```python
from build123d import *

# Parameters (mm, degrees)
SKETCH_2_R          = 1.75
SKETCH_2_R_2        = 6
EXTRUDE_1_DEPTH     = 8
SKETCH_3_R          = 8.05
CUT_EXTRUDE_1_DEPTH = 3.5
SKETCH_4_W          = 16.75
SKETCH_4_H          = 17
EXTRUDE_2_DEPTH     = 30
SKETCH_5_R          = 1.75
CUT_EXTRUDE_2_DEPTH = 51.685920136
EXTRUDE_3_DEPTH     = 2
EXTRUDE_4_DEPTH     = 2


with BuildPart() as part:
    # 草图2 → 凸台-拉伸1 (new body)
    with BuildSketch(Plane.XY):
        with BuildLine():
            Line((-6.25, 21.25), (6.25, 21.25))
            ThreePointArc((6.25, 21.25), (9.785533906, 19.785533906), (11.25, 16.25))
            Line((11.25, 16.25), (11.25, -16.25))
            ThreePointArc((11.25, -16.25), (9.785533906, -19.785533906), (6.25, -21.25))
            Line((6.25, -21.25), (-6.25, -21.25))
            ThreePointArc((-6.25, -21.25), (-9.785533906, -19.785533906), (-11.25, -16.25))
            Line((-11.25, -16.25), (-11.25, 16.25))
            ThreePointArc((-11.25, 16.25), (-9.785533906, 19.785533906), (-6.25, 21.25))
        make_face()
        with Locations((0, -16.25)):
            Circle(SKETCH_2_R, mode=Mode.SUBTRACT)
        Circle(SKETCH_2_R_2, mode=Mode.SUBTRACT)
        with Locations((0, 16.25)):
            Circle(SKETCH_2_R, mode=Mode.SUBTRACT)
    extrude(amount=EXTRUDE_1_DEPTH)

    # 草图3 → 切除-拉伸1 (cut)
    with BuildSketch(Plane(origin=(0, 0, 0), x_dir=(-1, 0, 0), z_dir=(0, 0, -1))):
        Circle(SKETCH_3_R)
    extrude(amount=-CUT_EXTRUDE_1_DEPTH, mode=Mode.SUBTRACT)

    # 草图4 → 凸台-拉伸2 (add)
    with BuildSketch(Plane.XY):
        with Locations((-19.625, 0)):
            Rectangle(SKETCH_4_W, SKETCH_4_H)
    extrude(amount=EXTRUDE_2_DEPTH)

    # 草图5 → 切除-拉伸2 (cut, through all)
    with BuildSketch(Plane.XZ.offset(8.5)):
        with Locations(Location((-23, 22.5, 0), (0, 0, 270))):
            Circle(SKETCH_5_R)
        with Locations(Location((-23, 7.5, 0), (0, 0, 270))):
            Circle(SKETCH_5_R)
    extrude(amount=-CUT_EXTRUDE_2_DEPTH, mode=Mode.SUBTRACT)

    # 草图7 → 凸台-拉伸3 (add)
    with BuildSketch(Plane.XZ.offset(8.5)):
        Polygon((-11.25, 20), (-11.25, 8), (-4.32179677, 8), align=None)
    extrude(amount=-EXTRUDE_3_DEPTH)

    # 草图8 → 凸台-拉伸4 (add)
    with BuildSketch(Plane(origin=(0, 8.5, 0), x_dir=(1, 0, 0), z_dir=(0, 1, 0))):
        Polygon((-4.32179677, -8), (-11.25, -20), (-11.25, -8), align=None)
    extrude(amount=-EXTRUDE_4_DEPTH)


solid = part.part
```
Can you work these out from the model? Positions are in its coordinate system, mm. A direction names the side the tool comes from. Coordinates: 2 decimals unless noted, no trailing zeros. Write each loop counter-clockwise with the first axis right and the second up, starting at its lowest first coordinate (ties: lowest second). Pieces come first, ordered by that corner, then holes. Notation, with made-up numbers: M 84.5,28 L 138.5,28 A20 cw 138.5,33 Z; hole C 80.25,74.5 d11. An arc over 180 degrees is marked long. Answer as CSV lines item,"result".
Item 1: Imagine slicing it at B-B on y = 0. List the corners of the cut face in (x, z) for me, plus the area to 3 significant figures.
Geometry results:
outline,"M -28,0 L -8.05,0 L -8.05,3.5 L -6,3.5 L -6,8 L -11.25,8 L -11.25,30 L -28,30 Z; M 6,3.5 L 8.05,3.5 L 8.05,0 L 11.25,0 L 11.25,8 L 6,8 Z; hole C -23,7.5 d3.5; hole C -23,22.5 d3.5"
area,"553 mm2"
Item 2: Please list where these lines run through material, in increasing order: line 1 along Y through (x, z) = (0, 6); line 2 along Y through (x, z) = (0, 3.25); line 3 along X through (y, z) = (3.25, 7.5).
Geometry results:
line 1,"y = -21.25 to -18, -14.5 to -6, 6 to 14.5, 18 to 21.25"
line 2,"y = -21.25 to -18, -14.5 to -8.05, 8.05 to 14.5, 18 to 21.25"
line 3,"x = -28 to -24.75, -21.25 to -5.04, 5.04 to 11.25"
Item 3: I'm going to push flat-ended pins straight in: P1, Ø3.5, axis at x = -7.5, z = 11, coming from the +Y side; P2, Ø13.5, axis at y = 1, z = 24, coming from the +X side; P3, Ø4, axis at x = 0, y = -16.25, coming from the +Z side. Where does each tip first touch, or does it pass through?
Geometry results:
P1,"stops at y = 8.5"
P2,"stops at x = -11.25"
P3,"stops at z = 8"
Item 4: Imagine slicing it at C-C on z = 22.5. List the corners of the cut face in (x, y) for me, plus the area to 3 significant figures.
Geometry results:
outline,"M -28,-8.5 L -24.75,-8.5 L -24.75,8.5 L -28,8.5 Z; M -21.25,-8.5 L -11.25,-8.5 L -11.25,8.5 L -21.25,8.5 Z"
area,"225 mm2"
Item 5: We'd pull the mould along Y, two halves only. Please class faces 1 (the flat face through (0, -21.25, 4)), 2 (the cylindrical face through (-6, 0, 6)), 3 (the cylindrical face through (9.75, 19.82, 3.94)): +Y half, -Y half, draft (parallel to the pull), parting line (faces both ways), or undercut.
Geometry results:
face 1,"-Y half"
face 2,"undercut"
face 3,"+Y half"
Item 6: Imagine slicing it at A-A on x = 0. List the corners of the cut face in (y, z) for me.
Geometry results:
outline,"M -21.25,0 L -18,0 L -18,8 L -21.25,8 Z; M -14.5,0 L -8.05,0 L -8.05,3.5 L -6,3.5 L -6,8 L -14.5,8 Z; M 6,3.5 L 8.05,3.5 L 8.05,0 L 14.5,0 L 14.5,8 L 6,8 Z; M 18,0 L 21.25,0 L 21.25,8 L 18,8 Z"
Item 7: Imagine slicing it at D-D on x = -23. List the corners of the cut face in (y, z) for me.
Geometry results:
outline,"M -8.5,0 L 8.5,0 L 8.5,5.75 L -8.5,5.75 Z; M -8.5,9.25 L 8.5,9.25 L 8.5,20.75 L -8.5,20.75 Z; M -8.5,24.25 L 8.5,24.25 L 8.5,30 L -8.5,30 Z"
Item 8: On a 3-axis mill with a long thin cutter (end or side, diameter ignored), from which of +Z, -Z, +X, -X, +Y, -Y can I reach the whole of each face in a straight line? I mean faces 4 (the cylindrical face through (-7.678, 2.418, 1.726)), 5 (the flat face through (-11.25, 12, 4)), 6 (the flat face through (-11.25, -12, 4)). Say none if no direction works.
Geometry results:
face 4,"-Z"
face 5,"+Z, -Z, -X, +Y"
face 6,"+Z, -Z, -X, -Y"
